Input: part model. Units: mm. Frame: model coordinates. Face numbers are marked on the shaded views. A direction names the side the tool comes from. Coordinates: 2 decimals unless noted, no trailing zeros. Order: outer loops, then holes, each group sorted by start corner. A loop starts at its lowest first (then second) coordinate and runs counter-clockwise, first axis right, second up.
from build123d import *

# Parameters (mm, degrees)
HOLE_WIZARD_8_2_8_2_1_D = 8.2


with BuildPart() as part:
    # Эскиз1 → Повернуть1 (revolve)
    with BuildSketch(Plane.XY):
        Polygon((1.2, 0), (1.2, 7.5), (8.2, 7.5), (8.2, 9.833333333), (10.2, 9.833333333), (10.2, 12.5), (43.5, 12.5), (43.5, 0), align=None)
    revolve(axis=Axis((-1000, 0, 0), (1, 0, 0)))

    # Диаметр отверстия Ø8.2 (8.2)1 (through all)
    with Locations(Plane.ZY.offset(-1.2)):
        with Locations((0, 0)):
            Hole(HOLE_WIZARD_8_2_8_2_1_D / 2)


solid = part.part
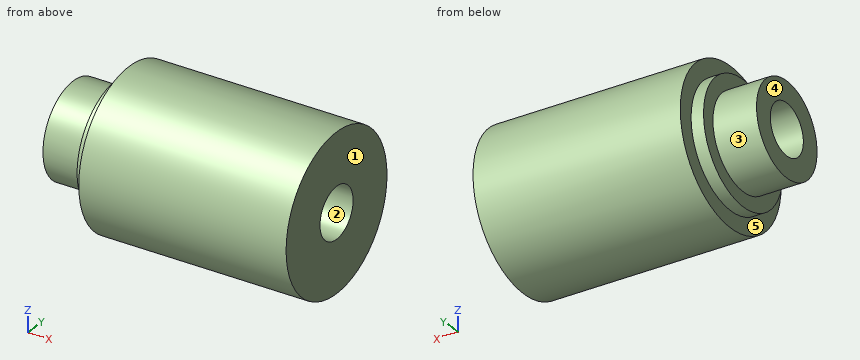
Item 1: Cut plane A-A on z = 0. Return loops of the section in (x, y), then the cut area to 3 significant figures.
Response values:
outline: (1.2, -7.5) - (8.2, -7.5) - (8.2, -9.83) - (10.2, -9.83) - (10.2, -12.5) - (43.5, -12.5) - (43.5, -4.1) - (1.2, -4.1) - close; (1.2, 4.1) - (43.5, 4.1) - (43.5, 12.5) - (10.2, 12.5) - (10.2, 9.83) - (8.2, 9.83) - (8.2, 7.5) - (1.2, 7.5) - close
area: 630 mm2
Item 2: Ray query, probe 1 along Z at (x, y) = (23, -1); probe 2 along X at (y, z) = (8.25, -6.5); probe 3 along X at (y, z) = (-6.5, 5.5). Return the intervals inside material, ascending.
Response values:
probe 1: z = -12.46 to -3.98, 3.98 to 12.46
probe 2: x = 10.2 to 43.5
probe 3: x = 8.2 to 43.5
Item 3: Access query for the marked faces 4 and 5. Directions: +Z, -Z, +X, -X, +Y, -Y. A direction counts if a zero-diameter tool reaches every point of the face in a straight line with its end or side. Return the directions, or none.
Response values:
face 4: +Z, -Z, -X, +Y, -Y
face 5: -X
Item 4: Cut plane C-C on x = 34.5. Return loops of the section in (y, z).
Response values:
outline: circle Ø25 at (0, 0); hole circle Ø8.2 at (0, 0)
Item 5: Draft query along Z for the marked faces 1, 2 and 3. Return one class per face: pulls with the +Z half, pulls with the -Z half, needs draft (parallel to the pull), parting line crosses it, or undercut.
Response values:
face 1: needs draft
face 2: undercut
face 3: parting line crosses it
Item 6: Cut plane D-D on z = -9.25. Return loops of the section in (x, y).
Response values:
outline: (8.2, -3.34) - (10.2, -3.34) - (10.2, -8.41) - (43.5, -8.41) - (43.5, 8.41) - (10.2, 8.41) - (10.2, 3.34) - (8.2, 3.34) - close
Item 7: Pin query (flat end, axial travel): pin 1 Ø1 at (y, z) = (-4.5, 9.5) entering from -X; pin 2 Ø1 at (x, y) = (13.5, 4) entering from -Z; pin 3 Ø1.5 at (y, z) = (9.5, 9.5) entering from +X; pin 4 Ø1.5 at (x, y) = (25, 10) entering from +Z. Return the tip coordinate at first contact, or that it passes through.
Response values:
pin 1: stops at x = 10.2
pin 2: stops at z = -12
pin 3: passes through
pin 4: stops at z = 8.41
